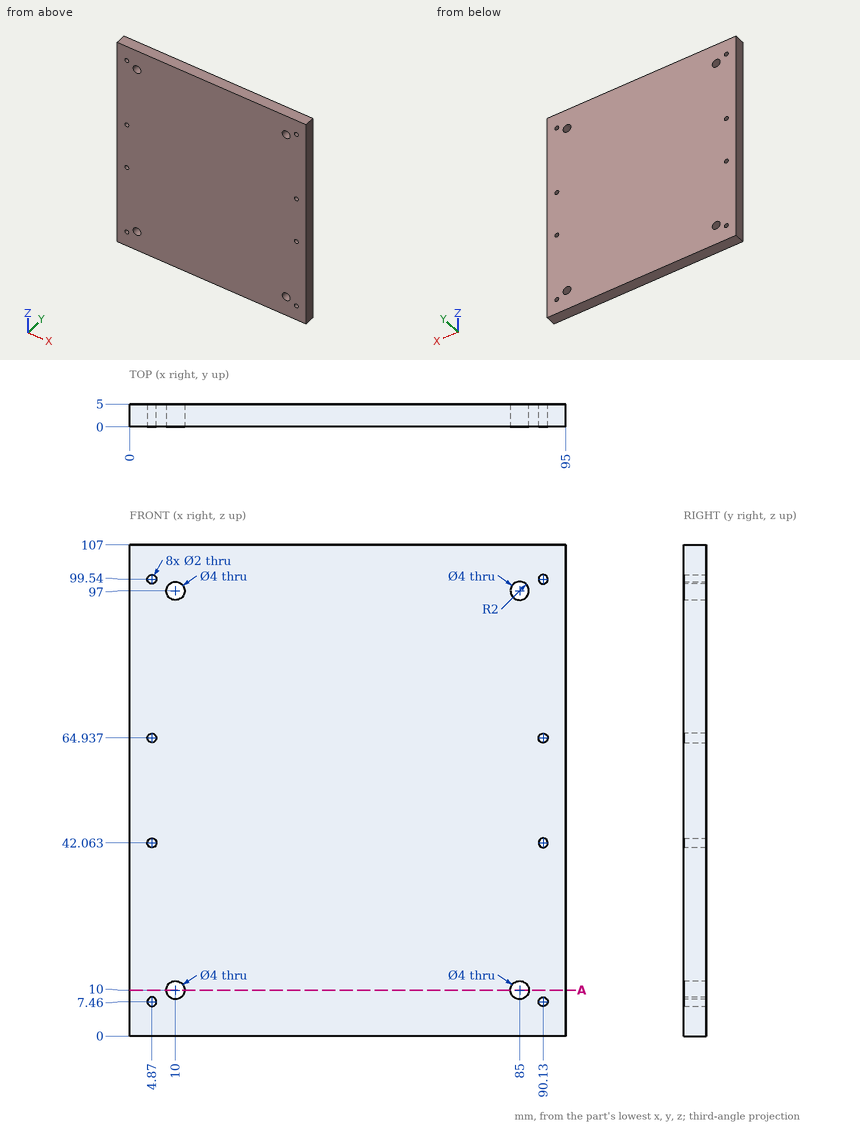
Job drawing, mm, ordinate dimensions from the low corner. One solid piece. Give positions to 0.01 mm unless a question says otherwise; leave off trailing zeros. Order: outer loops, then holes, each group sorted by start corner. A loop starts at its lowest first (then second) coordinate and runs counter-clockwise, first axis right, second up. Notation, with made-up numbers: M 70.5,68.25 L 94.5,68.25 A24 cw 94.5,106.25 Z; hole C 52,6 d3. An arc over 180 degrees is marked long. Put each result on its own line as item: value. Start each with the question number.
(1) Band-saw the part on A-A on z = 10. Give the cut face in (x, y), then the cut area to 3 significant figures.
(2) Pin check, flat tips, straight feed: pin 1 Ø2.5 at (x, z) = (90.13, 64.94) entering from +Y; pin 2 Ø1.6 at (x, z) = (90.13, 99.54) entering from +Y. Stop position of each tip, or through.
(3) Drill centre lines: L1, parallel to Z at x = 4.87, y = 3.4; L2, parallel to X at y = 2.1, z = 99.54. Where is each one in solid material? Low to high. Write a range as [from, to].
Results below:
1. outline: M 0,0 L 8,0 L 8,5 L 0,5 Z; M 12,0 L 83,0 L 83,5 L 12,5 Z; M 87,0 L 95,0 L 95,5 L 87,5 Z
1. area: 435 mm2
2. pin 1: stops at y = 5
2. pin 2: passes through
3. L1: z = [0, 6.46], [8.46, 41.06], [43.06, 63.94], [65.94, 98.54], [100.54, 107]
3. L2: x = [0, 3.87], [5.87, 89.13], [91.13, 95]
